Could you check a few things on this model? Use its own coordinates, in mm. A direction names the side the tool comes from. Coordinates: 2 decimals unless noted, no trailing zeros. Write each loop counter-clockwise with the first axis right and the second up, starting at its lowest first coordinate (ties: lowest second). Pieces come first, ordered by that corner, then holes.
Item 1: Thinking about a two-plate mould opening in Y: for faces 1 (the cylindrical face through (15.565, 2.479, 0.175)), 2 (the cylindrical face through (-15.64, 2.56, 0.18)), 3 (the cylindrical face through (-7.17, 14.04, 0.18)), 4 (the flat face through (-4, -10, -12.5)), which applies, +Y half, -Y half, draft (parallel to the pull), parting line (faces both ways), or undercut?
Item 2: I want a section at A-A on y = -6.5. Please give me the cut outline in (x, z).
Item 3: I want a section at C-C on y = 14. Please give me the cut outline in (x, z).
Item 4: If I drill on probe 1 along X at (y, z) = (12.5, -7.25); probe 2 along Y at (x, z) = (-12, 4.5); probe 3 along X at (y, z) = (-3, 9.75), over which ranges is the centre line in solid material (lowest first)?
Item 5: I want a section at B-B on x = 8. Please give me the cut outline in (y, z), then the cut area to 3 significant figures.
Item 6: Which directions (+Z, -Z, +X, -X, +Y, -Y) give clear straight access to the entire face, cutting with the end or side of a thin tool? Please do faces 5 (the cylindrical face through (-15.565, -2.479, 0.175)), 6 (the cylindrical face through (7.3, 14.1, 0.2)), 7 (the cylindrical face through (7.17, -14.04, 0.18)).
Item 7: For P1, Ø1, axis at x = 13, z = 0.5, coming from the +Y side; P2, Ø4, axis at x = 13, y = -9.5, coming from the -Z side; P3, Ø6, axis at x = 11.5, y = -9.5, coming from the -Z side; P4, Ø12, axis at x = 2, z = -2, coming from the +Y side, each with a flat end and sliding along its axis, tell me the tip position at first contact or that it passes through.
from build123d import *

# Parameters (mm, degrees)
BOSS_EXTRUDE1_DEPTH = 12.5
SKETCH2_R           = 10
CUT_EXTRUDE1_DEPTH  = 36.746855524


with BuildPart() as part:
    # Sketch1 → Boss-Extrude1 (new, symmetric)
    with BuildSketch(Plane.XY):
        with BuildLine():
            ThreePointArc((0, 18.51446423), (-2.427307325, 15.616232504), (-3.522517853, 11.9979343))
            ThreePointArc((-3.522517853, 11.9979343), (-3.586020803, 11.708984719), (-3.718536081, 11.444477279))
            ThreePointArc((-3.718536081, 11.444477279), (-3.981216766, 11.580577767), (-4.202432033, 11.777016791))
            ThreePointArc((-4.202432033, 11.777016791), (-7.215258285, 14.060532932), (-10.882529029, 14.978516204))
            ThreePointArc((-10.882529029, 14.978516204), (-11.142724039, 11.207062035), (-9.901985646, 7.636048701))
            ThreePointArc((-9.901985646, 7.636048701), (-9.783520309, 7.364957483), (-9.735253849, 7.073075942))
            ThreePointArc((-9.735253849, 7.073075942), (-10.027764846, 7.028783717), (-10.322195719, 7.057679154))
            ThreePointArc((-10.322195719, 7.057679154), (-14.101840469, 7.13418768), (-17.608301852, 5.721284089))
            ThreePointArc((-17.608301852, 5.721284089), (-15.601998897, 2.517174783), (-12.499231478, 0.357452038))
            ThreePointArc((-12.499231478, 0.357452038), (-12.244047587, 0.207766813), (-12.033435535, 0))
            ThreePointArc((-12.033435535, 0), (-12.244047587, -0.207766813), (-12.499231478, -0.357452038))
            ThreePointArc((-12.499231478, -0.357452038), (-15.601998897, -2.517174783), (-17.608301852, -5.721284089))
            ThreePointArc((-17.608301852, -5.721284089), (-14.101840469, -7.13418768), (-10.322195719, -7.057679154))
            ThreePointArc((-10.322195719, -7.057679154), (-10.027764846, -7.028783717), (-9.735253849, -7.073075942))
            ThreePointArc((-9.735253849, -7.073075942), (-9.783520309, -7.364957483), (-9.901985646, -7.636048701))
            ThreePointArc((-9.901985646, -7.636048701), (-11.142724039, -11.207062035), (-10.882529029, -14.978516204))
            ThreePointArc((-10.882529029, -14.978516204), (-7.215258285, -14.060532932), (-4.202432033, -11.777016791))
            ThreePointArc((-4.202432033, -11.777016791), (-3.981216766, -11.580577767), (-3.718536081, -11.444477279))
            ThreePointArc((-3.718536081, -11.444477279), (-3.586020803, -11.708984719), (-3.522517853, -11.9979343))
            ThreePointArc((-3.522517853, -11.9979343), (-2.427307325, -15.616232504), (0, -18.51446423))
            ThreePointArc((0, -18.51446423), (2.427307325, -15.616232504), (3.522517853, -11.9979343))
            ThreePointArc((3.522517853, -11.9979343), (3.586020803, -11.708984719), (3.718536081, -11.444477279))
            ThreePointArc((3.718536081, -11.444477279), (3.981216766, -11.580577767), (4.202432033, -11.777016791))
            ThreePointArc((4.202432033, -11.777016791), (7.215258285, -14.060532932), (10.882529029, -14.978516204))
            ThreePointArc((10.882529029, -14.978516204), (11.142724039, -11.207062035), (9.901985646, -7.636048701))
            ThreePointArc((9.901985646, -7.636048701), (9.783520309, -7.364957483), (9.735253849, -7.073075942))
            ThreePointArc((9.735253849, -7.073075942), (10.027764846, -7.028783717), (10.322195719, -7.057679154))
            ThreePointArc((10.322195719, -7.057679154), (14.101840469, -7.13418768), (17.608301852, -5.721284089))
            ThreePointArc((17.608301852, -5.721284089), (15.601998897, -2.517174783), (12.499231478, -0.357452038))
            ThreePointArc((12.499231478, -0.357452038), (12.244047587, -0.207766813), (12.033435535, 0))
            ThreePointArc((12.033435535, 0), (12.244047587, 0.207766813), (12.499231478, 0.357452038))
            ThreePointArc((12.499231478, 0.357452038), (15.601998897, 2.517174783), (17.608301852, 5.721284089))
            ThreePointArc((17.608301852, 5.721284089), (14.101840469, 7.13418768), (10.322195719, 7.057679154))
            ThreePointArc((10.322195719, 7.057679154), (10.027764846, 7.028783717), (9.735253849, 7.073075942))
            ThreePointArc((9.735253849, 7.073075942), (9.783520309, 7.364957483), (9.901985646, 7.636048701))
            ThreePointArc((9.901985646, 7.636048701), (11.142724039, 11.207062035), (10.882529029, 14.978516204))
            ThreePointArc((10.882529029, 14.978516204), (7.215258285, 14.060532932), (4.202432033, 11.777016791))
            ThreePointArc((4.202432033, 11.777016791), (3.981216766, 11.580577767), (3.718536081, 11.444477279))
            ThreePointArc((3.718536081, 11.444477279), (3.586020803, 11.708984719), (3.522517853, 11.9979343))
            ThreePointArc((3.522517853, 11.9979343), (2.427307325, 15.616232504), (0, 18.51446423))
        make_face()
    extrude(amount=BOSS_EXTRUDE1_DEPTH, both=True)

    # Sketch2 → Cut-Extrude1 (cut, through all)
    with BuildSketch(Plane.XY.offset(12.5)):
        Circle(SKETCH2_R)
    extrude(amount=-CUT_EXTRUDE1_DEPTH, mode=Mode.SUBTRACT)


solid = part.part
Response values:
1. face 1: undercut
1. face 2: undercut
1. face 3: +Y half
1. face 4: draft
2. outline: (-16.18, -12.5) - (-7.6, -12.5) - (-7.6, 12.5) - (-16.18, 12.5) - close; (7.6, -12.5) - (16.18, -12.5) - (16.18, 12.5) - (7.6, 12.5) - close
3. outline: (-11.1, -12.5) - (-7.09, -12.5) - (-7.09, 12.5) - (-11.1, 12.5) - close; (-3.12, -12.5) - (3.12, -12.5) - (3.12, 12.5) - (-3.12, 12.5) - close; (7.09, -12.5) - (11.1, -12.5) - (11.1, 12.5) - (7.09, 12.5) - close
4. probe 1: x = -11.23 to -4.91, -3.46 to 3.46, 4.91 to 11.23
4. probe 2: y = -7.28 to 7.28
4. probe 3: x = -16.03 to -9.54, 9.54 to 16.03
5. outline: (-14.39, -12.5) - (-6, -12.5) - (-6, 12.5) - (-14.39, 12.5) - close; (6, -12.5) - (14.39, -12.5) - (14.39, 12.5) - (6, 12.5) - close
5. area: 420 mm2
6. face 5: +Z, -Z, -X
6. face 6: +Z, -Z, +Y
6. face 7: +Z, -Z, -Y
7. P1: stops at y = 7.29
7. P2: passes through
7. P3: stops at z = -12.5
7. P4: stops at y = 18.51
